from build123d import *

# Parameters (mm, degrees)
SKETCH1_R          = 50.8
EXTRUDE1_DEPTH     = 320
FILLET1_R          = 25.4
SKETCH3_W          = 10
SKETCH3_H          = 20
CUT_EXTRUDE1_DEPTH = 7.62
SKETCH4_R          = 19.05
CUT_EXTRUDE2_DEPTH = 2.54


with BuildPart() as part:
    # Sketch1 → Extrude1 (new body)
    with BuildSketch(Plane(origin=(0, 0, 0), x_dir=(1, 0, 0), z_dir=(0, 1, 0))):
        with Locations(Location((0, 0, 0), (0, 0, 270))):
            Circle(SKETCH1_R)
    extrude(amount=EXTRUDE1_DEPTH)

    # Fillet1
    fillet1_edges = [part.edges().sort_by_distance(p)[0] for p in [
        (0, 0, -50.8),
        (0, 320, -50.8),
    ]]
    fillet(fillet1_edges, radius=FILLET1_R)

    # Sketch3 → Cut-Extrude1 (cut)
    with BuildSketch(Plane(origin=(0, 320, 0), x_dir=(1, 0, 0), z_dir=(0, 1, 0))):
        Rectangle(SKETCH3_W, SKETCH3_H)
    extrude(amount=-CUT_EXTRUDE1_DEPTH, mode=Mode.SUBTRACT)

    # Sketch4 → Cut-Extrude2 (cut)
    with BuildSketch(Plane.XZ):
        with Locations(Location((0, 0, 0), (0, 0, 270))):
            Circle(SKETCH4_R)
    extrude(amount=-CUT_EXTRUDE2_DEPTH, mode=Mode.SUBTRACT)


solid = part.part
Geometry: final body of the model. Coordinates: model frame, mm. A direction names the side the tool comes from. Round coordinates to 2 decimals unless told otherwise and drop trailing zeros. Loops run counter-clockwise (first coordinate to the right, second up) from the corner with the lowest first, then second, coordinate; pieces in that order, holes last.
Q1. Access query for faces 1 (the cylindrical face through (-11.59, 1.25, 15.12)), 2 (the flat face through (0, 316, 10)), 3 (the flat face through (19, 0, 4)). Directions: +Z, -Z, +X, -X, +Y, -Y. A direction counts if a zero-diameter tool reaches every point of the face in a straight line with its end or side. Return the directions, or none.
Q2. Pin query (flat end, axial travel): P1, Ø4, axis at x = 2, y = 317.5, coming from the +Z side; P2, Ø8, axis at x = 2, z = 3.5, coming from the -Y side; P3, Ø1.5, axis at y = 208, z = -26, coming from the -X side. Return the tip coordinate at first contact, or that it passes through.
Q3. Section A-A on y = 111.5. Return loops of the section in (x, z), plus the area to 3 significant figures.
Q4. Pull-direction query (X, two-part tool) for faces 4 (the flat face through (-5.3, 320, -0.4)), 5 (the cylindrical face through (-30.911, 158.116, -40.313)), 6 (the flat face through (0, 312.38, 0)); classes: released by +X, released by -X, zero draft, split by the parting line, or undercut.
Q5. Material intervals for L1, parallel to Z at x = -23, y = 20.5; L2, parallel to Y at x = -4, z = 44; L3, parallel to X at y = 269, z = 33.5, sorted ascending.
Evaluation:
1. face 1: -Y
1. face 2: +Y
1. face 3: +Z, -Z, +X, -X, -Y
2. P1: stops at z = 39.79
2. P2: stops at y = 2.54
2. P3: stops at x = -44.08
3. outline: circle Ø101.6 at (0, 0)
3. area: 8,110 mm2
4. face 4: zero draft
4. face 5: split by the parting line
4. face 6: undercut
5. L1: z = -44.76 to 44.76
5. L2: y = 8.3 to 311.7
5. L3: x = -38.19 to 38.19
